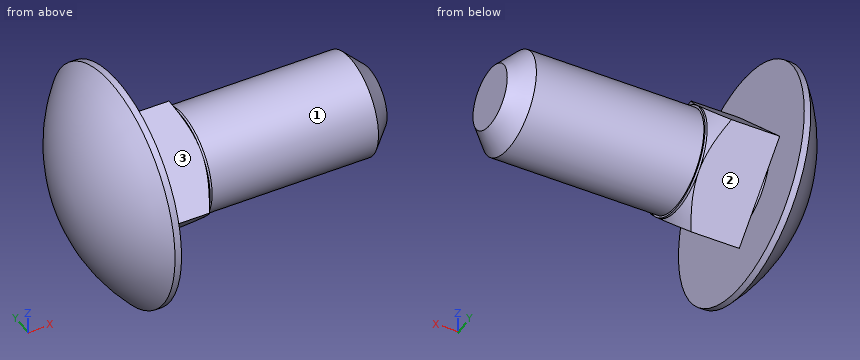
from build123d import *

# Parameters (mm, degrees)
EXTRUDE_START       = 0.1
EXTRUDE_1_DEPTH     = 2.9
SKETCH_6_R          = 2.5
SKETCH_6_R_2        = 2.4
CUT_EXTRUDE_1_DEPTH = 8.9


with BuildPart() as part:
    # Эскиз3 → Повернуть1 (revolve)
    with BuildSketch(Plane.XY):
        with BuildLine():
            Line((12, 0), (12, 1.5))
            Line((12, 1.5), (11, 2.5))
            Line((11, 2.5), (0, 2.5))
            Line((0, 2.5), (0, 5.5))
            Line((0, 5.5), (-0.309475019, 5.5))
            ThreePointArc((-0.309475019, 5.5), (-1.9322204, 2.960084445), (-2.5, 0))
            Line((-2.5, 0), (12, 0))
        make_face()
    revolve(axis=Axis((-123.766149148, 0, 0), (1, 0, 0)))

    # Эскиз4 → Бобышка-Вытянуть1 (add)
    with BuildSketch(Plane(origin=(0, 0, 0), x_dir=(0, 0, -1), z_dir=(1, 0, 0)).offset(EXTRUDE_START)):
        Polygon((0, 3.535533906), (-3.535533906, 0), (0, -3.535533906), (3.535533906, 0), align=None)
    extrude(amount=EXTRUDE_1_DEPTH)


with BuildPart() as body_2:
    # Эскиз5 → Повернуть2 (revolve)
    with BuildSketch(Plane.XY):
        Polygon((3, 2.5), (2.402134221, 3.535533906), (3, 3.535533906), align=None)
    revolve(axis=Axis((-123.766149148, 0, 0), (1, 0, 0)))


with BuildPart() as part_1:
    add(part.part)

    # Combine 1: cut body 2
    add(body_2.part, mode=Mode.SUBTRACT)

    # Эскиз6 → Вырез-Вытянуть1 (cut)
    with BuildSketch(Plane(origin=(12, 0, 0), x_dir=(0, 0, -1), z_dir=(1, 0, 0))):
        Circle(SKETCH_6_R)
        Circle(SKETCH_6_R_2, mode=Mode.SUBTRACT)
    extrude(amount=-CUT_EXTRUDE_1_DEPTH, mode=Mode.SUBTRACT)


solid = part_1.part
CAD build for the part. Positions are in the model's coordinates, mm. Face numbers are marked on the shaded views. A direction names the side the tool comes from. Give positions to 0.01 mm unless a question says otherwise; leave off trailing zeros. Order: outer loops, then holes, each group sorted by start corner. A loop starts at its lowest first (then second) coordinate and runs counter-clockwise, first axis right, second up. Notation, with made-up numbers: (57.25, 21) - (86.25, 21) arc R29 cw to (86.25, 42) - close; hole circle Ø10 at (-38.5, 32.5). An arc over 180 degrees is marked (long way). Write each question's results on one line, items separated by ' | '.
1. Probe L1, parallel to X at y = -2.5, z = 4.25; L2, parallel to Z at x = 7.75, y = 1.5; L3, parallel to X at y = 0.25, z = -0.25. List the from-to ranges inside material, lowest first. Write a range as from..to.
Calculated:
L1: x = -0.8..0 | L2: z = -1.87..1.87 | L3: x = -2.49..12
2. 3-axis set-ups, long thin cutter, end or side, ignore diameter. For the marked faces 1, 2 and 3: which of +Z, -Z, +X, -X, +Y, -Y reach the whole face in a straight line?
Calculated:
face 1: +X | face 2: -Z, +X, +Y | face 3: +Z, +X, -Y
3. Saw through at B-B on x = 4. List the corners of the cut face in (y, z), and give its area (3 significant figures).
Calculated:
outline: circle Ø4.8 at (0, 0) | area: 18.1 mm2
4. Pin check, flat tips, straight feed: pin 1 (1.9 mm diameter, centred on y = 2.5, z = 0.5, fed in from -X); pin 2 (1.5 mm diameter, centred on x = 10.5, y = 1.5, fed in from -Z); pin 3 (6 mm diameter, centred on x = 5, z = 0.5, fed in from -Y). Stop position of each tip, or through.
Calculated:
pin 1: stops at x = -2.34 | pin 2: stops at z = -2.28 | pin 3: stops at y = -3.54
5. Saw through at A-A on z = -3.75. List the corners of the cut face in (x, y).
Calculated:
outline: (-0.31, -4.02) - (0, -4.02) - (0, 4.02) - (-0.31, 4.02) arc R7.07 ccw to start
6. Saw through at C-C on z = 4. List the corners of the cut face in (x, y), and give its area (4 significant figures).
Calculated:
outline: (-0.31, -3.77) - (0, -3.77) - (0, 3.77) - (-0.31, 3.77) arc R6.93 ccw to start | area: 8.065 mm2
